Source: three-view drawing plus pictorial views. Frame: mm from the lowest corner of the part. Give positions to 0.01 mm unless a question says otherwise; leave off trailing zeros. Loops run counter-clockwise (first coordinate to the right, second up) from the corner with the lowest first, then second, coordinate; pieces in that order, holes last. Notation, with made-up numbers: (31.5, 76.5) -> (86.5, 76.5) arc R28 cw to (86.5, 111.5) -> close; hole circle Ø10 at (12, 61). An arc over 180 degrees is marked (long way). Answer as a JSON object with one key per item and string values. Group by question number.
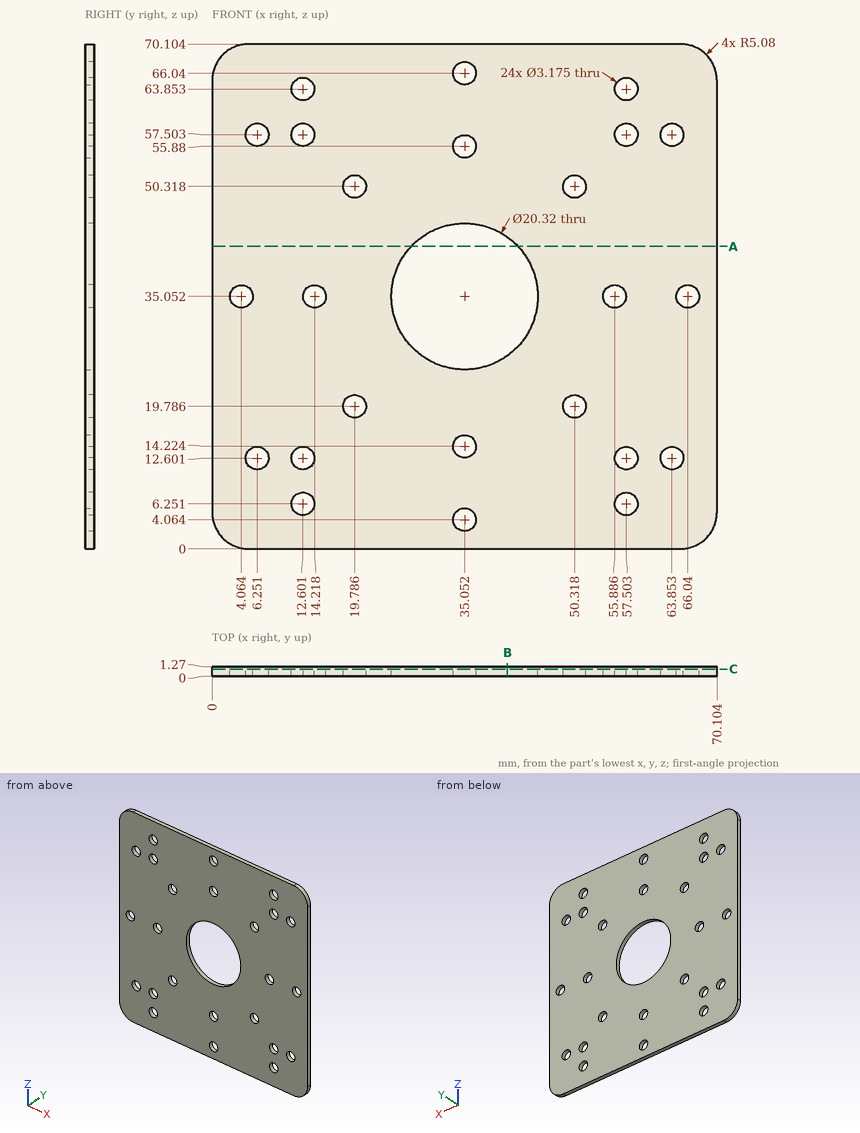
(1) Section query C-C on y = 0.95. State how many separate pieces and enclosed holes the cut face has, plus the area to 3 significant figures.
(2) Material intervals for line 1 (X direction, y = 0.7, z = 19.5) (1 decimal); line 2 (Z direction, x = 12.5, y = 0.65) (1 decimal); line 3 (X direction, y = 1.1, z = 62.5) (1 decimal), sorted ascending. Write a range as from..to.
(3) Section query A-A on z = 42. Return the cut outline in (x, y) (1 decimal).
(4) First-contact query: pin 1 (5 mm diameter, centred on x = 4.064, z = 35.052, fed in from -Y); pin 2 (1.9 mm diameter, centred on x = 12.6, z = 6.25, fed in from -Y). Flat tips, straight axial feed; report the tip coordinate or a pass-through.
(5) Section query B-B on x = 41. Return the cut outline in (y, z) (1 decimal).
Result:
{
 "1": {"separate pieces": "1", "enclosed holes": "25", "area": "4,380 mm²"},
 "2": {"line 1": "0..18.2, 21.3..48.8, 51.9..70.1", "line 2": "0..4.7, 7.8..11, 14.2..55.9, 59.1..62.3, 65.4..70.1", "line 3": "0..11.8, 13.4..56.7, 58.3..70.1"},
 "3": {"outline": "(0, 0) -> (27.6, 0) -> (27.6, 1.3) -> (0, 1.3) -> close; (42.5, 0) -> (70.1, 0) -> (70.1, 1.3) -> (42.5, 1.3) -> close"},
 "4": {"pin 1": "y = 0", "pin 2": "through"},
 "5": {"outline": "(0, 0) -> (1.3, 0) -> (1.3, 26.8) -> (0, 26.8) -> close; (0, 43.3) -> (1.3, 43.3) -> (1.3, 70.1) -> (0, 70.1) -> close"}
}
